Source: three-view drawing plus pictorial views. Frame: mm from the lowest corner of the part. A direction names the side the tool comes from. Round coordinates to 2 decimals unless told otherwise and drop trailing zeros. Loops run counter-clockwise (first coordinate to the right, second up) from the corner with the lowest first, then second, coordinate; pieces in that order, holes last. Notation, with made-up numbers: M 84.5,87 L 142.5,87 A6 ccw 142.5,96 Z; hole C -28.5,-15 d2. An arc over 180 degrees is marked long. Answer as a JSON object with one key per item and string values.
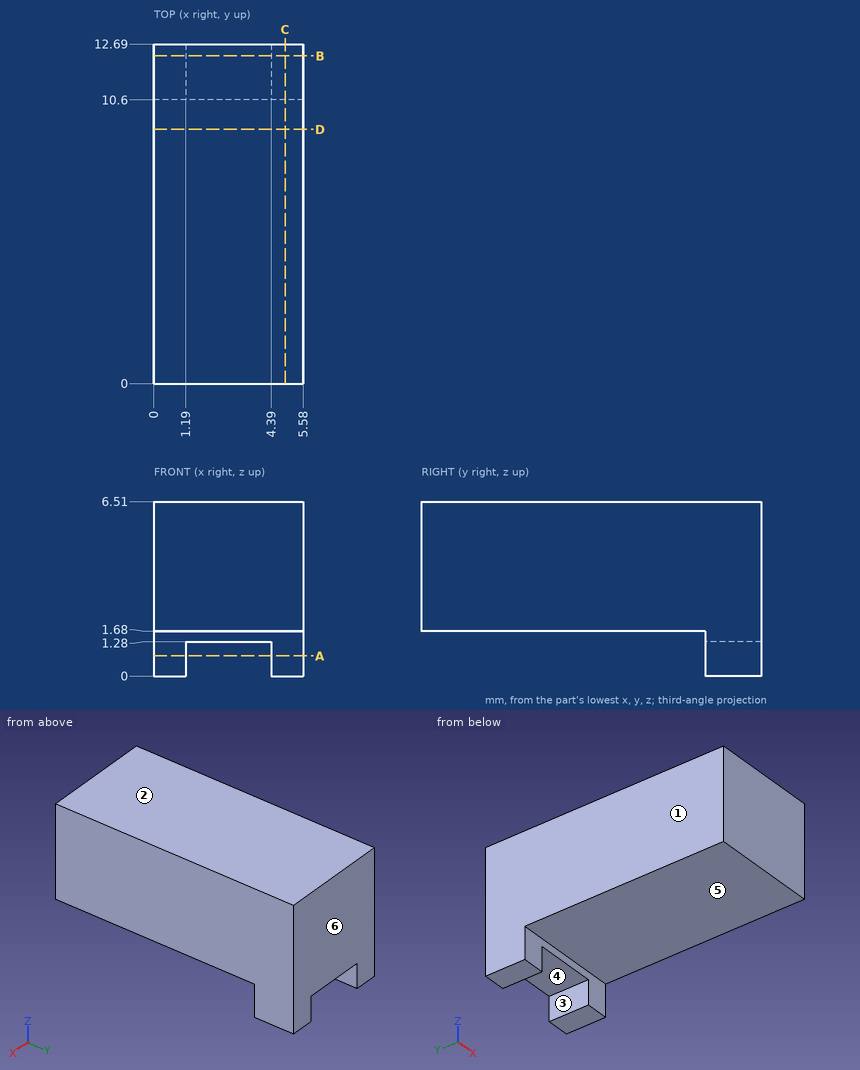
1) Cut plane B-B on y = 12.25. Return the cut outline in (x, z).
Geometry results:
{"outline": "M 0,0 L 1.19,0 L 1.19,1.28 L 4.39,1.28 L 4.39,0 L 5.58,0 L 5.58,6.51 L 0,6.51 Z"}
2) First-contact query: pin 1 (2 mm diameter, centred on y = 1.5, z = 3.5, fed in from -X); pin 2 (0.6 mm diameter, centred on x = 2, y = 11.5, fed in from -Z); pin 3 (2 mm diameter, centred on x = 3.5, y = 5, fed in from -Z). Flat tips, straight axial feed; report the tip coordinate or a pass-through.
Geometry results:
{"pin 1": "x = 0", "pin 2": "z = 1.28", "pin 3": "z = 1.68"}
3) Set-up query: the marked faces 4, 5 and 6. Return all of +Z, -Z, +X, -X, +Y, -Y with unobstructed straight access to the full face (end or side cutting, diameter ignored); none if empty.
Geometry results:
{"face 4": "-Z, +Y, -Y", "face 5": "-Z, +X, -X, -Y", "face 6": "+Z, -Z, +X, -X, +Y"}
4) Cut plane C-C on x = 4.9. Return the cut outline in (y, z), and give its area (3 significant figures).
Geometry results:
{"outline": "M 0,1.68 L 10.6,1.68 L 10.6,0 L 12.69,0 L 12.69,6.51 L 0,6.51 Z", "area": "64.8 mm2"}
5) Cut plane D-D on y = 9.5. Return the cut outline in (x, z), and give its area (3 significant figures).
Geometry results:
{"outline": "M 0,1.68 L 5.58,1.68 L 5.58,6.51 L 0,6.51 Z", "area": "27.0 mm2"}
6) Pull-direction query (X, two-part tool) for the marked faces 1, 2 and 3; classes: +X half, -X half, draft (parallel to the pull), parting line (faces both ways), or undercut.
Geometry results:
{"face 1": "-X half", "face 2": "draft", "face 3": "undercut"}
7) Line query: probe 1 along Z at (x, y) = (1.55, 1); probe 2 along Z at (x, y) = (3.35, 11.25); probe 3 along Y at (x, z) = (5.2, 1.5). Output: solid intervals per line, ascending.
Geometry results:
{"probe 1": "1.68 to 6.51", "probe 2": "1.28 to 6.51", "probe 3": "10.6 to 12.69"}
8) Cut plane A-A on z = 0.75. Return the cut outline in (x, y).
Geometry results:
{"outline": "M 0,10.6 L 1.19,10.6 L 1.19,12.69 L 0,12.69 Z; M 4.39,10.6 L 5.58,10.6 L 5.58,12.69 L 4.39,12.69 Z"}
